from build123d import *

# Parameters (mm, degrees)
F1_DEPTH  = 3
F4_DEPTH  = 3.5
F5_R      = 4
F6_DEPTH  = 2
F8_DEPTH  = 3.5
F9_R      = 4
F10_DEPTH = 2


with BuildPart() as f1:
    # F0 (on Front) → F1 (new body)
    with BuildSketch(Plane.XZ):
        with BuildLine():
            Line((42.3408785927, 7.5), (40.3081877539, 7.5))
            ThreePointArc((40.3081877539, 7.5), (40.6920731694, -5.0154941107), (37.2806551355, -17.0631987819))
            Line((37.2806551355, -17.0631987819), (39.4695736908, -17.0631987819))
            ThreePointArc((39.4695736908, -17.0631987819), (42.7091934986, -4.9924734046), (42.3408785927, 7.5))
        make_face()
    extrude(amount=F1_DEPTH)

    # F2: F1 across plane


with BuildPart() as f1_1:
    add(f1.part)
    add(f1.part.mirror(Plane.XZ))

    # F3 (on face) → F4 (join)
    with BuildSketch(Plane.XZ.offset(3)):
        with BuildLine():
            ThreePointArc((37.2806551355, -17.0631987819), (22.151849245, -34.5006605013), (0, -41))
            Line((0, -41), (0, -43))
            ThreePointArc((0, -43), (23.6144283477, -35.9354807093), (39.4695736908, -17.0631987819))
            Line((39.4695736908, -17.0631987819), (37.2806551355, -17.0631987819))
        make_face()
        with BuildLine():
            Line((42.3408785927, 7.5), (40.3081877539, 7.5))
            ThreePointArc((40.3081877539, 7.5), (40.6920731694, -5.0154941107), (37.2806551355, -17.0631987819))
            Line((37.2806551355, -17.0631987819), (39.4695736908, -17.0631987819))
            ThreePointArc((39.4695736908, -17.0631987819), (42.7091934986, -4.9924734046), (42.3408785927, 7.5))
        make_face()
    extrude(amount=F4_DEPTH)

    # F5 (on face) → F6 (join)
    with BuildSketch(Plane.XZ.offset(6.5)):
        with BuildLine():
            ThreePointArc((36.5205421647, -7.5), (38.9170857283, -8.6954006131), (39.4037428619, -11.3289473684))
            ThreePointArc((39.4037428619, -11.3289473684), (40.9527782079, -1.9672206414), (40.3082103224, 7.4998787062))
            Line((40.3082103224, 7.4998787062), (-0.1951071863, 7.4974617829))
            ThreePointArc((-0.1951071863, 7.4974617829), (-7.4993654189, -0.0975618479), (0, -7.5))
            Line((0, -7.5), (36.5205421647, -7.5))
        make_face()
        Circle(F5_R, mode=Mode.SUBTRACT)
        with BuildLine():
            ThreePointArc((39.4037428619, -11.3289473684), (38.4492475072, -14.2357074334), (37.2806551355, -17.0631987819))
            ThreePointArc((37.2806551355, -17.0631987819), (22.151849245, -34.5006605013), (0, -41))
            Line((0, -41), (0, -43))
            ThreePointArc((0, -43), (23.6144283477, -35.9354807093), (39.4695736908, -17.0631987819))
            ThreePointArc((39.4695736908, -17.0631987819), (42.7091934986, -4.9924734046), (42.3408785927, 7.5))
            Line((42.3408785927, 7.5), (40.3082103224, 7.4998787062))
            ThreePointArc((40.3082103224, 7.4998787062), (40.9527782079, -1.9672206414), (39.4037428619, -11.3289473684))
        make_face()
    extrude(amount=F6_DEPTH)

    # F7 (on face) → F8 (join)
    with BuildSketch(Plane(origin=(0, 3, 0), x_dir=(-1, 0, 0), z_dir=(0, 1, 0))):
        with BuildLine():
            Line((-40.3081877539, 7.5), (-42.3408785927, 7.5))
            Line((-42.3408785927, 7.5), (-42.3578410098, 7.4036008123))
            ThreePointArc((-42.3578410098, 7.4036008123), (-42.7034836956, -5.0410792753), (-39.4695736908, -17.0631987819))
            Line((-39.4695736908, -17.0631987819), (-37.2806551355, -17.0631987819))
            ThreePointArc((-37.2806551355, -17.0631987819), (-40.6920731694, -5.0154941107), (-40.3081877539, 7.5))
        make_face()
        with BuildLine():
            ThreePointArc((-17.9295521431, -36.8718206758), (-29.3280944194, -28.6507046637), (-37.2806551355, -17.0631987819))
            Line((-37.2806551355, -17.0631987819), (-39.4695736908, -17.0631987819))
            ThreePointArc((-39.4695736908, -17.0631987819), (-31.2153660392, -29.5736525143), (-19.1686619835, -38.491069065))
            Line((-19.1686619835, -38.491069065), (-17.9295521431, -36.8718206758))
        make_face()
    extrude(amount=F8_DEPTH)

    # F9 (on face) → F10 (join)
    with BuildSketch(Plane(origin=(0, 6.5, 0), x_dir=(-1, 0, 0), z_dir=(0, 1, 0))):
        with BuildLine():
            Line((0.0050283843, 7.4999983144), (-40.3081877539, 7.5))
            ThreePointArc((-40.3081877539, 7.5), (-40.9528037605, -1.9666886256), (-39.4040031085, -11.3280421532))
            ThreePointArc((-39.4040031085, -11.3280421532), (-38.9173062041, -8.6945341056), (-36.5207833689, -7.4991610201))
            Line((-36.5207833689, -7.4991610201), (0.1121784082, -7.4991610201))
            ThreePointArc((0.1121784082, -7.4991610201), (7.4998086337, 0.0535766476), (0.0050283843, 7.4999983144))
        make_face()
        Circle(F9_R, mode=Mode.SUBTRACT)
        with BuildLine():
            Line((-40.3081877539, 7.5), (-42.3408785927, 7.5))
            Line((-42.3408785927, 7.5), (-42.3578410098, 7.4036008123))
            ThreePointArc((-42.3578410098, 7.4036008123), (-38.3791326561, -19.3918069444), (-19.1686619835, -38.491069065))
            Line((-19.1686619835, -38.491069065), (-17.9295521431, -36.8718206758))
            ThreePointArc((-17.9295521431, -36.8718206758), (-31.3832008366, -26.3836067521), (-39.4040031085, -11.3280421532))
            ThreePointArc((-39.4040031085, -11.3280421532), (-40.9528037605, -1.9666886256), (-40.3081877539, 7.5))
        make_face()
    extrude(amount=F10_DEPTH)


solid = f1_1.part
Check sheet for the modelled part. Datum: model origin and axes. Units: mm. A direction names the side the tool comes from. Coordinates: 2 decimals unless noted, no trailing zeros. Write each loop counter-clockwise with the first axis right and the second up, starting at its lowest first coordinate (ties: lowest second). Pieces come first, ordered by that corner, then holes.
Item 1: Access from +Z, -Z, +X, -X, +Y, -Y to the whole of each face (thin tool, end or side, straight path). Record for faces 1 (the face through (38, 0, -17.063)), 2 (the face through (18, 7, -7.499)), 3 (the face through (0, -6, -42)).
Numbers:
face 1: -Z, +X, -X
face 2: -X, +Y, -Y
face 3: -Z, -X, +Y, -Y
Item 2: Cross-section at D-D on x = 20.5. Record the boundary of the cut face in (y, z).
Numbers:
outline: (-8.5, -37.8) - (-3, -37.8) - (-3, -35.51) - (-8.5, -35.51) - close; (-8.5, -7.5) - (-6.5, -7.5) - (-6.5, 7.5) - (-8.5, 7.5) - close; (3, -37.8) - (8.5, -37.8) - (8.5, -35.51) - (3, -35.51) - close; (6.5, -7.5) - (8.5, -7.5) - (8.5, 7.5) - (6.5, 7.5) - close
Item 3: Cross-section at C-C on y = -7.5. Record the boundary of the cut face in (x, z).
Numbers:
outline: (-0.2, 7.5) arc R7.5 ccw to (0, -7.5) - (36.52, -7.5) arc R3 cw to (39.4, -11.33) arc R41 cw to (0, -41) - (0, -43) arc R43 ccw to (42.34, 7.5) - close; hole circle Ø8 at (0, 0)
Item 4: Scan lines: probe 1 along Y at (x, z) = (25, 1.5); probe 2 along Z at (x, y) = (0, 7.05); probe 3 along X at (y, z) = (5.5, -1). Record each from-to range of solid material in increasing order.
Numbers:
probe 1: y = -8.5 to -6.5, 6.5 to 8.5
probe 2: z = -7.5 to -4, 4 to 7.5
probe 3: x = 40.99 to 42.99
Item 5: Cross-section at B-B on x = 38.5. Record the boundary of the cut face in (y, z).
Numbers:
outline: (-8.5, -19.15) - (-3, -19.15) - (-3, -17.06) - (3, -17.06) - (3, -19.15) - (8.5, -19.15) - (8.5, -14.1) - (-8.5, -14.1) - close; (-8.5, -8.25) - (-6.5, -8.25) - (-6.5, 7.5) - (-8.5, 7.5) - close; (6.5, -8.24) - (8.5, -8.24) - (8.5, 7.5) - (6.5, 7.5) - close
Item 6: Mould release check, pull along Z, two halves, no side actions. Record for faces 4 (the face through (22, 8.5, -2)), 5 (the face through (18, -7, -7.5)), 6 (the face through (18.558, 5.712, -37.693)), 7 (the face through (38.94, 7.486, -8.726)): released by +Z, released by -Z, zero draft, split by the parting line, or undercut.
Numbers:
face 4: zero draft
face 5: undercut
face 6: released by -Z
face 7: undercut
Item 7: Cross-section at A-A on z = 0. Record the boundary of the cut face in (x, y), then the cut area to 3 significant figures.
Numbers:
outline: (-7.5, -8.5) - (-4, -8.5) - (-4, -6.5) - (-7.5, -6.5) - close; (-7.5, 6.5) - (-4, 6.5) - (-4, 8.5) - (-7.5, 8.5) - close; (4, -8.5) - (43, -8.5) - (43, 8.5) - (4, 8.5) - (4, 6.5) - (41, 6.5) - (41, -6.5) - (4, -6.5) - close
area: 196 mm2
Item 8: Depth check by flat-ended pin: pin 1 Ø1.6 at (x, y) = (25.5, 7.5) entering from -Z; pin 2 Ø1 at (y, z) = (6.5, -24) entering from -X; pin 3 Ø8 at (y, z) = (6, -37.5) entering from +X; pin 4 Ø4 at (x, z) = (11.5, -10.5) entering from +Y. Enter the tip coordinate at first touch or a pass-through.
Numbers:
pin 1: stops at z = -35.2
pin 2: stops at x = 32.87
pin 3: stops at x = 26.96
pin 4: passes through
